```python
from build123d import *

# Parameters (mm, degrees)
F1_DEPTH = 5
F2_R     = 3.925
F3_DEPTH = 5.001
F4_R     = 2
F5_R     = 1


with BuildPart() as f1:
    # F0 (on Front) → F1 (new body)
    with BuildSketch(Plane.XZ):
        with BuildLine():
            ThreePointArc((22.5, 30.5), (0, 8), (-22.5, 30.5))
            Line((-22.5, 30.5), (-22.5, 48))
            Line((-22.5, 48), (-25.2045257213, 48))
            ThreePointArc((-25.2045257213, 48), (-29, 43.075), (-32.7954742787, 48))
            Line((-32.7954742787, 48), (-35.5, 48))
            Line((-35.5, 48), (-35.5, 0))
            Line((-35.5, 0), (35.5, 0))
            Line((35.5, 0), (35.5, 48))
            Line((35.5, 48), (32.7954742787, 48))
            ThreePointArc((32.7954742787, 48), (29, 43.075), (25.2045257213, 48))
            Line((25.2045257213, 48), (22.5, 48))
            Line((22.5, 48), (22.5, 30.5))
        make_face()
    extrude(amount=F1_DEPTH)

    # F2 (on Front) → F3 (cut, through all)
    with BuildSketch(Plane.XZ):
        with Locations((-28, 3.725)):
            Circle(F2_R)
        with Locations((28, 3.725)):
            Circle(F2_R)
    extrude(amount=F3_DEPTH, mode=Mode.SUBTRACT)

    # F4
    f4_edges = [f1.edges().sort_by_distance(p)[0] for p in [
        (-22.5, -2.5, 48),
        (22.5, -2.5, 48),
        (-35.5, -2.5, 48),
        (35.5, -2.5, 48),
        (35.5, -2.5, 0),
        (-35.5, -2.5, 0),
    ]]
    fillet(f4_edges, radius=F4_R)

    # F5
    f5_edges = [f1.edges().sort_by_distance(p)[0] for p in [
        (-26.763068, -2.5, 0),
        (-29.236932, -2.5, 0),
        (29.236932, -2.5, 0),
        (26.763068, -2.5, 0),
    ]]
    fillet(f5_edges, radius=F5_R)


solid = f1.part
```
The listing builds one solid part. Answer for the finished solid, in the listing's coordinates (mm). A direction names the side the tool comes from. Give positions to 0.01 mm unless a question says otherwise; leave off trailing zeros. Order: outer loops, then holes, each group sorted by start corner. A loop starts at its lowest first (then second) coordinate and runs counter-clockwise, first axis right, second up. Notation, with made-up numbers: (56, 0) -> (98, 0) arc R11 cw to (98, 11) -> close; hole circle Ø5 at (9, -5.5). An arc over 180 degrees is marked (long way). One line per item, written item: value.
1) A tool of negligible diameter and unlimited length cuts with its end or side. For faces 1 (the cylindrical face through (-31.23, -2.46, 0.51)), 2 (the flat face through (-22.5, -2, 38)), 3 (the flat face through (0, -2, 0)), from which of +Z, -Z, +X, -X, +Y, -Y can it reach the whole face along a straight path? Write none if from no direction.
Reported:
face 1: +Y, -Y
face 2: +Z, +Y, -Y
face 3: -Z, +X, -X, +Y, -Y
2) Determine the mould class of faces 4 (the cylindrical face through (-23.1, -2.54, 47.43)), 5 (the cylindrical face through (34.93, -2.54, 0.6)), 6 (the cylindrical face through (-24.77, -2.46, 0.51)) for opening direction Z: pulls with the +Z half, pulls with the -Z half, needs draft (parallel to the pull), parting line crosses it, or undercut.
Reported:
face 4: pulls with the +Z half
face 5: pulls with the -Z half
face 6: undercut
3) Find section A-A, the plane z = 41.5. Determine the outline of the cut face in (x, y), plus the area to 3 significant figures.
Reported:
outline: (-35.5, -5) -> (-22.5, -5) -> (-22.5, 0) -> (-35.5, 0) -> close; (22.5, -5) -> (35.5, -5) -> (35.5, 0) -> (22.5, 0) -> close
area: 130 mm^2
4) Flat-ended cylindrical pins translate along their axes: P1, Ø12.5, axis at x = 28, z = 3.725, coming from the -Y side; P2, Ø4.5, axis at x = 29, z = 47, coming from the +Y side. Find the tip coordinate at first contact, or state that the pin passes through.
Reported:
P1: stops at y = -5
P2: passes through
5) Find section D-D, the plane z = 47. Determine the outline of the cut face in (x, y) (3 decimals).
Reported:
outline: (-35.232, -5) -> (-32.925, -5) -> (-32.925, 0) -> (-35.232, 0) -> close; (-25.075, -5) -> (-22.768, -5) -> (-22.768, 0) -> (-25.075, 0) -> close; (22.768, -5) -> (25.075, -5) -> (25.075, 0) -> (22.768, 0) -> close; (32.925, -5) -> (35.232, -5) -> (35.232, 0) -> (32.925, 0) -> close
6) Find section B-B, the plane y = -0.9. Determine the outline of the cut face in (x, z) (3 decimals), plus the area to 3 significant figures.
Reported:
outline: (-35.5, 2) arc R2 ccw to (-33.5, 0) -> (-32.102, 0) arc R1 ccw to (-31.269, 1.553) arc R3.925 cw (long way) to (-24.731, 1.553) arc R1 ccw to (-23.898, 0) -> (23.898, 0) arc R1 ccw to (24.731, 1.553) arc R3.925 cw (long way) to (31.269, 1.553) arc R1 ccw to (32.102, 0) -> (33.5, 0) arc R2 ccw to (35.5, 2) -> (35.5, 46) arc R2 ccw to (33.5, 48) -> (32.795, 48) arc R3.925 cw (long way) to (25.205, 48) -> (24.5, 48) arc R2 ccw to (22.5, 46) -> (22.5, 30.5) arc R22.5 cw to (-22.5, 30.5) -> (-22.5, 46) arc R2 ccw to (-24.5, 48) -> (-25.205, 48) arc R3.925 cw (long way) to (-32.795, 48) -> (-33.5, 48) arc R2 ccw to (-35.5, 46) -> close
area: 1,660 mm^2
7) Find the intervals of material crossed by line 1 (X direction, y = -1.6, z = 47) (3 decimals); line 2 (X direction, y = -4.55, z = 40); line 3 (X direction, y = -3.3, z = 2), in increasing order.
Reported:
line 1: x = -35.232 to -32.925, -25.075 to -22.768, 22.768 to 25.075, 32.925 to 35.232
line 2: x = -35.5 to -22.5, 22.5 to 35.5
line 3: x = -35.5 to -31.53, -24.47 to 24.47, 31.53 to 35.5
8) Find section C-C, the plane z = 16. Determine the outline of the cut face in (x, y), plus the area to 3 significant figures.
Reported:
outline: (-35.5, -5) -> (-17.2, -5) -> (-17.2, 0) -> (-35.5, 0) -> close; (17.2, -5) -> (35.5, -5) -> (35.5, 0) -> (17.2, 0) -> close
area: 183 mm^2
